Verification items for the finished model (mm, model axes). Give positions to 0.01 mm unless a question says otherwise; leave off trailing zeros. Write each loop counter-clockwise with the first axis right and the second up, starting at its lowest first coordinate (ties: lowest second). Pieces come first, ordered by that corner, then holes. Notation, with made-up numbers: (-1.5, -8.75) -> (46.5, -8.75) arc R7 ccw to (46.5, 0.25) -> close; hole circle Ø11 at (27, 26.5). An arc over 180 degrees is marked (long way). Write item = value, one per line.
from build123d import *

# Parameters (mm, degrees)
CROQUIS2_W                   = 220
CROQUIS2_H                   = 220
CROQUIS2_W_2                 = 200
CROQUIS2_H_2                 = 200
SALIENTE_EXTRUIR1_DEPTH      = 10
CROQUIS3_W                   = 212
CROQUIS3_H                   = 212
CROQUIS3_W_2                 = 210
CROQUIS3_H_2                 = 210
CROQUIS3_W_3                 = 208
CROQUIS3_H_3                 = 208
CORTAR_EXTRUIR1_DEPTH        = 3.5
CROQUIS4_W                   = 10
CROQUIS4_H                   = 10
SALIENTE_EXTRUIR2_DEPTH      = 200
SALIENTE_EXTRUIR2_DEPTH_BACK = 10
CROQUIS6_W                   = 3.5
CROQUIS6_H                   = 2
CROQUIS6_W_2                 = 2
CROQUIS6_H_2                 = 3.5
CROQUIS6_W_3                 = 1.99805467
CORTAR_EXTRUIR2_DEPTH        = 203.5
CROQUIS7_W                   = 220
CROQUIS7_H                   = 220
CROQUIS7_W_2                 = 200
CROQUIS7_H_2                 = 200
SALIENTE_EXTRUIR3_DEPTH      = 10
CORTAR_EXTRUIR3_START        = -3.5
CROQUIS8_W                   = 207
CROQUIS8_H                   = 2
CORTAR_EXTRUIR3_DEPTH        = 207
MATRIZC1_COUNT               = 4
CROQUIS9_W                   = 86
CROQUIS9_H                   = 16
BRAZOS_DEPTH                 = 10
MATRIZC2_COUNT               = 4
CROQUIS10_W                  = 237.555255491
CROQUIS10_H                  = 247.362549521
CORTAR_EXTRUIR4_DEPTH        = 221
CROQUIS11_W                  = 253.49457107
CROQUIS11_H                  = 258.277976667
CORTAR_EXTRUIR5_DEPTH        = 11
SALIENTE_EXTRUIR4_START      = -6
CROQUIS12_R                  = 2.8
SALIENTE_EXTRUIR4_DEPTH      = 16
CROQUIS13_R                  = 2.8
SALIENTE_EXTRUIR5_DEPTH      = 10
SALIENTE_EXTRUIR5_DEPTH_BACK = 10


with BuildPart() as part:
    # Croquis2 → Saliente-Extruir1 (new body)
    with BuildSketch(Plane.XY):
        with Locations((110, -110)):
            Rectangle(CROQUIS2_W, CROQUIS2_H)
        with Locations((110, -110)):
            Rectangle(CROQUIS2_W_2, CROQUIS2_H_2, mode=Mode.SUBTRACT)
    extrude(amount=SALIENTE_EXTRUIR1_DEPTH)

    # Croquis3 → Cortar-Extruir1 (cut)
    with BuildSketch(Plane.XY.offset(10)):
        with Locations((110, -110)):
            Rectangle(CROQUIS3_W, CROQUIS3_H)
        with Locations((110, -110)):
            Rectangle(CROQUIS3_W_2, CROQUIS3_H_2, mode=Mode.SUBTRACT)
        with Locations((110, -110)):
            Rectangle(CROQUIS3_W_2, CROQUIS3_H_2)
        with Locations((110, -110)):
            Rectangle(CROQUIS3_W_3, CROQUIS3_H_3, mode=Mode.SUBTRACT)
    extrude(amount=-CORTAR_EXTRUIR1_DEPTH, mode=Mode.SUBTRACT)

    # Croquis4 → Saliente-Extruir2 (add, two sides)
    with BuildSketch(Plane.XY.offset(10)) as saliente_extruir2_sk:
        with Locations((5, -5)):
            Rectangle(CROQUIS4_W, CROQUIS4_H)
        with Locations((215, -5)):
            Rectangle(CROQUIS4_W, CROQUIS4_H)
        with Locations((215, -215)):
            Rectangle(CROQUIS4_W, CROQUIS4_H)
        with Locations((5, -215)):
            Rectangle(CROQUIS4_W, CROQUIS4_H)
    extrude(amount=SALIENTE_EXTRUIR2_DEPTH)
    extrude(saliente_extruir2_sk.sketch, amount=-SALIENTE_EXTRUIR2_DEPTH_BACK)

    # Croquis6 → Cortar-Extruir2 (cut)
    with BuildSketch(Plane.XY.offset(210)):
        with Locations((8.25, -5)):
            Rectangle(CROQUIS6_W, CROQUIS6_H)
        with Locations((5, -8.25)):
            Rectangle(CROQUIS6_W_2, CROQUIS6_H_2)
        with Locations((211.75, -5)):
            Rectangle(CROQUIS6_W, CROQUIS6_H)
        with Locations((215, -8.25)):
            Rectangle(CROQUIS6_W_2, CROQUIS6_H_2)
        with Locations((211.75, -215)):
            Rectangle(CROQUIS6_W, CROQUIS6_H)
        with Locations((215.000972665, -211.75)):
            Rectangle(CROQUIS6_W_3, CROQUIS6_H_2)
        with Locations((5, -211.75)):
            Rectangle(CROQUIS6_W_2, CROQUIS6_H_2)
        with Locations((8.25, -215)):
            Rectangle(CROQUIS6_W, CROQUIS6_H)
    extrude(amount=-CORTAR_EXTRUIR2_DEPTH, mode=Mode.SUBTRACT)

    # Croquis7 → Saliente-Extruir3 (add)
    with BuildSketch(Plane.XY.offset(210)):
        with Locations((110, -110)):
            Rectangle(CROQUIS7_W, CROQUIS7_H)
        with Locations((110, -110)):
            Rectangle(CROQUIS7_W_2, CROQUIS7_H_2, mode=Mode.SUBTRACT)
    extrude(amount=SALIENTE_EXTRUIR3_DEPTH)

    # Croquis8 → Cortar-Extruir3 (cut)
    with BuildSketch(Plane(origin=(0, -210, 0), x_dir=(1, 0, 0), z_dir=(0, 1, 0)).offset(CORTAR_EXTRUIR3_START)):
        with Locations((110, -215)):
            Rectangle(CROQUIS8_W, CROQUIS8_H)
    cortar_extruir3 = extrude(amount=CORTAR_EXTRUIR3_DEPTH, mode=Mode.SUBTRACT)

    # MatrizC1: Cortar-Extruir3 ×4 about axis
    matrizc1_axis = Axis((0, -110, 110), (1, 0, 0))
    for i in range(1, MATRIZC1_COUNT):
        add(cortar_extruir3.rotate(matrizc1_axis, i * 360 / MATRIZC1_COUNT), mode=Mode.SUBTRACT)

    # Croquis9 → Brazos (add)
    with BuildSketch(Plane.XY.offset(220)):
        with Locations((43, -110)):
            Rectangle(CROQUIS9_W, CROQUIS9_H)
        with BuildLine():
            ThreePointArc((71.801526277, -112.25), (69.551526277, -110), (71.801526277, -107.75))
            Line((71.801526277, -107.75), (75, -107.75))
            ThreePointArc((75, -107.75), (77.25, -110), (75, -112.25))
            Line((75, -112.25), (71.801526277, -112.25))
        make_face(mode=Mode.SUBTRACT)
        with Locations((177, -110)):
            Rectangle(CROQUIS9_W, CROQUIS9_H)
        with BuildLine():
            Line((145, -107.75), (148.198473723, -107.75))
            ThreePointArc((148.198473723, -107.75), (150.448473723, -110), (148.198473723, -112.25))
            Line((148.198473723, -112.25), (145, -112.25))
            ThreePointArc((145, -112.25), (142.75, -110), (145, -107.75))
        make_face(mode=Mode.SUBTRACT)
    extrude(amount=-BRAZOS_DEPTH)

    # MatrizC2: Cortar-Extruir3 ×4 about axis
    matrizc2_axis = Axis((110, 0, 110), (0, 1, 0))
    for i in range(1, MATRIZC2_COUNT):
        add(cortar_extruir3.rotate(matrizc2_axis, i * 360 / MATRIZC2_COUNT), mode=Mode.SUBTRACT)

    # Croquis10 → Cortar-Extruir4 (cut, through all)
    with BuildSketch(Plane.ZY):
        with Locations((128.777627746, -111.472396129)):
            Rectangle(CROQUIS10_W, CROQUIS10_H)
    extrude(amount=-CORTAR_EXTRUIR4_DEPTH, mode=Mode.SUBTRACT)

    # Croquis11 → Cortar-Extruir5 (cut, through all)
    with BuildSketch(Plane.XY.offset(10)):
        with Locations((136.747285535, -106.715640527)):
            Rectangle(CROQUIS11_W, CROQUIS11_H)
    extrude(amount=-CORTAR_EXTRUIR5_DEPTH, mode=Mode.SUBTRACT)

    # Croquis12 → Saliente-Extruir4 (add)
    with BuildSketch(Plane.XY.offset(10).offset(SALIENTE_EXTRUIR4_START)):
        with Locations((5, -5)):
            Circle(CROQUIS12_R)
        with Locations((5, -215)):
            Circle(CROQUIS12_R)
    extrude(amount=SALIENTE_EXTRUIR4_DEPTH)

    # Croquis13 → Saliente-Extruir5 (add, two sides)
    with BuildSketch(Plane(origin=(10, 0, 0), x_dir=(0, 0, -1), z_dir=(1, 0, 0))) as saliente_extruir5_sk:
        with Locations((-5, -5)):
            Circle(CROQUIS13_R)
        with Locations((-5, -215)):
            Circle(CROQUIS13_R)
    extrude(amount=SALIENTE_EXTRUIR5_DEPTH)
    extrude(saliente_extruir5_sk.sketch, amount=-SALIENTE_EXTRUIR5_DEPTH_BACK)


solid = part.part
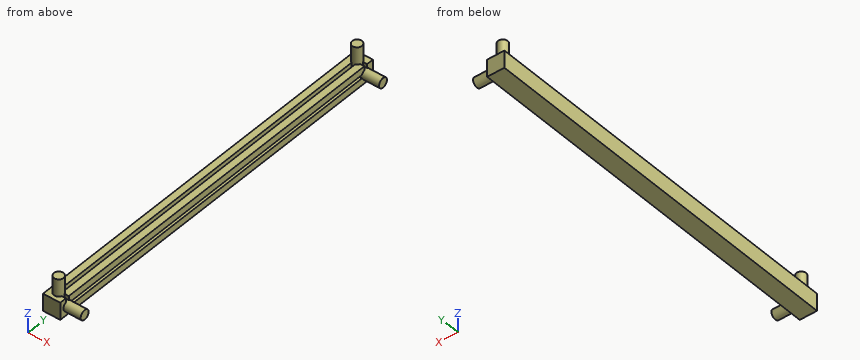
Item 1: Material ranges on line 1 (X direction, y = -181, z = 9.25); line 2 (Y direction, x = 4.5, z = 10.75) (3 decimals), recorded low to high.
Response values:
line_1 = 0 to 4, 6 to 10
line_2 = -217.755 to -212.245, -7.755 to -2.245
Item 2: Sectioned sample at B-B on x = 16.5. Record the cut outline in (y, z), then the cut area to 3 significant figures.
Response values:
outline = circle Ø5.6 at (-215, 5); circle Ø5.6 at (-5, 5)
area = 49.3 mm^2
Item 3: Sectioned sample at A-A on z = 14. Record the cut outline in (x, y).
Response values:
outline = circle Ø5.6 at (5, -215); circle Ø5.6 at (5, -5)
Item 4: Sectioned sample at C-C on y = -160. Record the cut outline in (x, z).
Response values:
outline = (0, 0) -> (10, 0) -> (10, 4) -> (6.5, 4) -> (6.5, 6) -> (10, 6) -> (10, 10) -> (6, 10) -> (6, 6.5) -> (4, 6.5) -> (4, 10) -> (0, 10) -> close
Item 5: Go/stop test with flat-tipped pins: P1, Ø5, axis at y = -162.5, z = 7, coming from the +X side; P2, Ø3, axis at x = 4.5, y = -64, coming from the +Z side; P3, Ø1, axis at x = 5, y = -60, coming from the +Z side. Record where each tip stops, or that it passes through.
Response values:
P1 = 10
P2 = 10
P3 = 6.5
